Source: CAD feature listing. Evaluate the final solid. Frame: model axes, mm. A direction names the side the tool comes from. Round coordinates to 2 decimals unless told otherwise and drop trailing zeros. Loops run counter-clockwise (first coordinate to the right, second up) from the corner with the lowest first, then second, coordinate; pieces in that order, holes last.
Item 1: Section query A-A on x = 0. Return loops of the section in (y, z), then the cut area to 3 significant figures.
Item 2: Ray query, L1, parallel to Z at x = 0, y = 31.5; L2, parallel to X at y = 25, z = 1.25; L3, parallel to Y at x = -2.25, z = 4.75. Return the intervals inside material, ascending.
Item 3: Pull-direction query (Z, two-part tool) for faces 3 (the cylindrical face through (2.17, 40.28, -9.76)), 4 (the cylindrical face through (-7.493, -64.93, 0.33)), 5 (the flat face through (0, 20, 0)), 6 (the flat face through (0, -70, 0)); classes: released by +Z, released by -Z, zero draft, split by the parting line, or undercut.
Item 4: Section query C-C on y = 45. Return loops of the section in (x, z), then the cut area to 3 significant figures.
Item 5: First-contact query: P1, Ø5, axis at x = -2, z = 2.5, coming from the +Y side. Flat tip, straight axial feed; report the tip coordinate or a pass-through.
Item 6: Section query B-B on z = 0. Return loops of the section in (x, y).
Item 7: Section query D-D on x = 12.75. Return loops of the section in (y, z).
Item 8: Access query for faces 1 (the flat face through (-4, -60, 7)), 2 (the flat face through (-0.2, 60, 10.2)). Directions: +Z, -Z, +X, -X, +Y, -Y. A direction counts if a zero-diameter tool reaches every point of the face in a straight line with its end or side. Return the directions, or none.
```python
from build123d import *

# Parameters (mm, degrees)
F1_DEPTH = 60
F2_R     = 7.5
F3_DEPTH = 10
F4_R     = 10
F5_DEPTH = 40


with BuildPart() as f1:
    # F0 (on Front) → F1 (new body, symmetric)
    with BuildSketch(Plane.XZ):
        Polygon((15, -15), (15, 0), (15, 15), (0, 15), (-15, 15), (-15, -15), align=None)
    extrude(amount=F1_DEPTH, both=True)

    # F2 (on face) → F3 (join)
    with BuildSketch(Plane.XZ.offset(60)):
        Circle(F2_R)
    extrude(amount=F3_DEPTH)

    # F4 (on face) → F5 (cut)
    with BuildSketch(Plane(origin=(0, 60, 0), x_dir=(-1, 0, 0), z_dir=(0, 1, 0))):
        Circle(F4_R)
    extrude(amount=-F5_DEPTH, mode=Mode.SUBTRACT)


solid = f1.part
```
Data:
1. outline: (-70, -7.5) - (-60, -7.5) - (-60, -15) - (60, -15) - (60, -10) - (20, -10) - (20, 10) - (60, 10) - (60, 15) - (-60, 15) - (-60, 7.5) - (-70, 7.5) - close
1. area: 2,950 mm2
2. L1: z = -15 to -10, 10 to 15
2. L2: x = -15 to -9.92, 9.92 to 15
2. L3: y = -70 to 20
3. face 3: undercut
3. face 4: split by the parting line
3. face 5: undercut
3. face 6: zero draft
4. outline: (-15, -15) - (15, -15) - (15, 15) - (-15, 15) - close; hole circle Ø20 at (0, 0)
4. area: 586 mm2
5. P1: stops at y = 20
6. outline: (-15, -60) - (-7.5, -60) - (-7.5, -70) - (7.5, -70) - (7.5, -60) - (15, -60) - (15, 60) - (10, 60) - (10, 20) - (-10, 20) - (-10, 60) - (-15, 60) - close
7. outline: (-60, -15) - (60, -15) - (60, 15) - (-60, 15) - close
8. face 1: -Y
8. face 2: +Z, -Z, +X, -X, +Y
